Work out the finished part from the listing and answer in its coordinate system (mm). A direction names the side the tool comes from. Give positions to 0.01 mm unless a question says otherwise; leave off trailing zeros. Write each loop counter-clockwise with the first axis right and the second up, starting at its lowest first coordinate (ties: lowest second). Pieces come first, ordered by that corner, then holes.
1) Given pin 1 Ø18.5 at (x, z) = (2.5, 5.5) entering from +Y; pin 2 Ø4 at (y, z) = (-3, 10) entering from -X; pin 3 Ø5 at (x, y) = (15.5, 4) entering from -Z, each flat-ended and moving along its own axis, determine where each tip first touches the part or whether it passes through.
2) Find section D-D (z = 14). Determine the outline of the cut face in (x, y), plus the area to 3 significant figures.
3) Find section B-B (x = 7). Determine the outline of the cut face in (y, z).
4) Determine the mould class of faces 1 (the face through (-10.382, 0.986, 19.961)), 2 (the face through (0, -6, 8.2)), 3 (the face through (-8, 2, -4)) for opening direction X: pulls with the +X half, pulls with the -X half, needs draft (parallel to the pull), parting line crosses it, or undercut.
5) Find section A-A (z = 0). Determine the outline of the cut face in (x, y).
6) Straight lines are drawn through the part: probe 1 along Z at (x, y) = (0, 4.1); probe 2 along X at (y, z) = (4.25, -0.5); probe 3 along Z at (x, y) = (0, 0.25). For each, find the intervals that lie inside material, in ascending order.
7) A tool of negligible diameter and unlimited length cuts with its end or side. For faces 4 (the face through (-9.9, 2, -18.2)), 5 (the face through (-2.17, -2.96, 9.76)), 6 (the face through (-1.73, -2.06, -7.81)), from which of +Z, -Z, +X, -X, +Y, -Y can it reach the whole face along a straight path? Write none if from no direction.
8) Find section C-C (x = -14). Determine the outline of the cut face in (y, z).
Autodesk Inventor part; units mm, degrees
ref_plane "YZ Plane" through (0, 0, 0) normal (1, 0, 0) x (0, 1, 0)
ref_plane "XZ Plane" through (0, 0, 0) normal (0, 1, 0) x (-1, 0, 0)
ref_plane "XY Plane" through (0, 0, 0) normal (0, 0, 1) x (1, 0, 0)
sketch "Sketch1" plane through (0, 0, 0) normal (0, 1, 0) x (-1, 0, 0)
  circle A0 centre (0, 0) radius 22.5
  dimension "d0" = 45
extrude "Extrusion1" add sketch "Sketch1" along normal blind 2
sketch "Sketch2" plane through (0, 2, 0) normal (0, 1, 0) x (1, 0, 0)
  circle A0 centre (0, 0) radius 22.5
  circle A1 centre (0, 0) radius 20.5
  circle A2 centre (0, 0) radius 18.5
  dimension "d3" = 2
  dimension "d4" = 4
extrude "Extrusion2" add sketch "Sketch2" along normal blind 5 contours A1
sketch "Sketch3" plane through (0, 0, 0) normal (0, -1, 0) x (1, 0, 0)
  circle A0 centre (0, 0) radius 20.5
  circle A1 centre (0, 0) radius 22.5
  circle A2 centre (0, 0) radius 8
  dimension "d7" = 16
extrude "Extrusion3" cut sketch "Sketch3" against normal blind 3 contours A2
sketch "Sketch4" plane through (0, 0, 0) normal (0, -1, 0) x (1, 0, 0)
  circle A0 centre (0, 0) radius 8
  circle A1 centre (0, 0) radius 22.5
  circle A2 centre (0, 0) radius 8
  circle A3 centre (0, 0) radius 10
  dimension "d10" = 2
extrude "Extrusion4" add sketch "Sketch4" along normal blind 6 contours A3
properties part number "Pieza 1.2 final" material "ABS Plastic"
Results:
1. pin 1: stops at y = 2
1. pin 2: stops at x = -6
1. pin 3: stops at z = -17.61
2. outline: (-17.61, 0) - (17.61, 0) - (17.61, 2) - (14.97, 2) - (14.97, 7) - (12.09, 7) - (12.09, 2) - (-12.09, 2) - (-12.09, 7) - (-14.97, 7) - (-14.97, 2) - (-17.61, 2) - close
2. area: 99.3 mm2
3. outline: (-6, -7.14) - (0, -7.14) - (0, -21.38) - (2, -21.38) - (2, -19.27) - (7, -19.27) - (7, -17.12) - (2, -17.12) - (2, -3.87) - (-6, -3.87) - close; (-6, 3.87) - (2, 3.87) - (2, 17.12) - (7, 17.12) - (7, 19.27) - (2, 19.27) - (2, 21.38) - (0, 21.38) - (0, 7.14) - (-6, 7.14) - close
4. face 1: parting line crosses it
4. face 2: needs draft
4. face 3: undercut
5. outline: (-22.5, 0) - (-10, 0) - (-10, -6) - (-8, -6) - (-8, 2) - (-18.5, 2) - (-18.5, 7) - (-20.5, 7) - (-20.5, 2) - (-22.5, 2) - close; (8, -6) - (10, -6) - (10, 0) - (22.5, 0) - (22.5, 2) - (20.5, 2) - (20.5, 7) - (18.5, 7) - (18.5, 2) - (8, 2) - close
6. probe 1: z = -20.5 to -18.5, 18.5 to 20.5
6. probe 2: x = -20.49 to -18.49, 18.49 to 20.49
6. probe 3: z = -22.5 to -8, 8 to 22.5
7. face 4: +Y
7. face 5: -Y
7. face 6: +Y, -Y
8. outline: (0, -17.61) - (2, -17.61) - (2, -14.97) - (7, -14.97) - (7, -12.09) - (2, -12.09) - (2, 12.09) - (7, 12.09) - (7, 14.97) - (2, 14.97) - (2, 17.61) - (0, 17.61) - close
